Autodesk Fusion 360 part; units mm, degrees
sketch "M3 Standoff Profile" plane through (0, 0, 0) normal (0, 1, 0) x (1, 0, 0)
  arc A0 (-2.75, -1.3669) -> (-2.5588, -1.6981) centre (-2.3675, -1.3669) ccw
  arc A1 (0.1912, 3.065) -> (-0.1913, 3.065) centre (0, 2.7338) ccw
  arc A2 (-0.1912, -3.065) -> (0.1913, -3.065) centre (0, -2.7338) ccw
  arc A3 (2.5588, -1.6981) -> (2.75, -1.3669) centre (2.3675, -1.3669) ccw
  line L0 (2.75, -1.3669) -> (2.75, 1.3669)
  line L1 (-2.75, 1.3669) -> (-2.75, -1.3669)
  arc A4 (2.75, 1.3669) -> (2.5588, 1.6981) centre (2.3675, 1.3669) ccw
  line L2 (-0.1913, 3.065) -> (-2.5588, 1.6981)
  line L3 (2.5587, 1.6981) -> (0.1912, 3.065)
  line L4 (-2.5588, -1.6981) -> (-0.1912, -3.065)
  line L5 (0.1913, -3.065) -> (2.5588, -1.6981)
  arc A5 (-2.5588, 1.6981) -> (-2.75, 1.3669) centre (-2.3675, 1.3669) ccw
  line L6 (0, 2.7338) -> (0, -2.7338) construction
  dimension "d28" = 120
  dimension "d29" = 0.3825
  dimension "d30" = 2.75
  dimension "d31" = 5.5
  dimension "d32" = 120
extrude "Extrude1" add sketch "M3 Standoff Profile" along normal blind 20
hole "Hole1" at (0, 0, 0) direction (0, 1, 0) diameter 2.529 depth 8 tip angle 118
ref_plane "WorkPlane1" through (0, 10, 0) normal (0.5, 0, 0.866) x (0.866, 0, -0.5)
sketch "Sketch2" plane through (0, 0, 0) normal (0.5, 0, 0.866) x (0.866, 0, -0.5)
  line L0 (-3.065, 0) -> (-1.6981, 0)
  line L1 (-1.6981, 0) -> (-1.6981, 20)
  line L2 (-1.6981, 20) -> (-3.065, 20)
  line L3 (-3.065, 20) -> (-3.065, 0)
  line L4 (1.6981, 0) -> (3.065, 0)
  line L5 (3.065, 20) -> (1.6981, 20)
  line L6 (1.6981, 20) -> (1.6981, 0)
  line L7 (-3.065, 0) -> (-3.1163, 0)
  line L8 (-3.065, 0) -> (-3.065, 20)
  line L9 (-3.065, 20) -> (-3.1163, 20)
  line L10 (-3.065, 20) -> (-3.065, 0)
  line L11 (3.1163, 0) -> (3.065, 0)
  line L12 (3.1163, 20) -> (3.065, 20)
  line L13 (3.065, 20) -> (3.065, 0) construction
  line L14 (1.6981, 0) -> (1.3669, 0)
  line L15 (1.6981, 0) -> (1.6981, 20)
  line L16 (1.6981, 20) -> (1.3669, 20)
  line L17 (1.3669, 20) -> (1.3669, 0)
  line L18 (3.1163, 0) -> (3.1163, 0.25)
  line L19 (3.1163, 0) -> (2.8663, 0)
  line L20 (2.8663, 0) -> (3.1163, 0.25)
  line L21 (3.1163, 20) -> (2.8663, 20)
  line L22 (3.1163, 20) -> (3.1163, 19.75)
  line L23 (2.8663, 20) -> (3.1163, 19.75)
  dimension "d12" = 0.25
  dimension "d13" = 0.25
  dimension "d14" = 0.25
  dimension "d15" = 0.25
revolve "Revolve1" cut sketch "Sketch2" angle 360 about axis through (0, 1.75, 0) along (0, 1, 0) contours L4 L11 L18 L19 L20 | L5 L12 L21 L22 L23
sketch "Sketch3" plane through (0, 20, 0) normal (0, 1, 0) x (-1, 0, 0)
  arc A0 (-0.6752, -2.7856) -> (0.6752, -2.7856) centre (0, 0) ccw
  line L0 (0.6752, -2.7856) -> (2.0748, -1.9776)
  arc A1 (2.0748, -1.9776) -> (2.75, -0.808) centre (0, 0) ccw
  line L1 (2.75, -0.808) -> (2.75, 0.808)
  arc A2 (2.75, 0.808) -> (2.0748, 1.9776) centre (0, 0) ccw
  line L2 (2.0748, 1.9776) -> (0.6752, 2.7856)
  arc A3 (0.6752, 2.7856) -> (-0.6752, 2.7856) centre (0, 0) ccw
  line L3 (-0.6752, 2.7856) -> (-2.0748, 1.9776)
  arc A4 (-2.0748, 1.9776) -> (-2.75, 0.808) centre (0, 0) ccw
  line L4 (-2.75, 0.808) -> (-2.75, -0.808)
  arc A5 (-2.75, -0.808) -> (-2.0748, -1.9776) centre (0, 0) ccw
  line L5 (-2.0748, -1.9776) -> (-0.6752, -2.7856)
  circle A6 centre (0, 0) radius 1.5
  circle A7 centre (0, 0) radius 1.35
  dimension "d17" = 3
  dimension "d18" = 2.7
extrude "Extrude2" add sketch "Sketch3" along normal blind 0.75 contours A7
extrude "Extrude3" add sketch "Sketch3" along normal blind 4 from surface at 0.75 contours A6 | A7
fillet "Fillet1" radius 0.25 1 edges at (1.2586, 20, 0.4882)
chamfer "Chamfer3" distance 0.15 angle 45 2 edges at (1.3985, 20.75, -0.5424) (1.3985, 24.75, -0.5424)
chamfer "Chamfer3" distance 0.3 angle 45 1 edges at (0.4573, 0, 1.1789)
equation "Thread_Length = 4 mm"
equation "Spacing = 20 mm"
equation "d3 = Spacing"
equation "d22 = Thread_Length"
equation "d30 = Hex_Width / 2"
equation "d31 = d30 * 2"
equation "d32 = d28"
equation "Hex_Width = 5.5 mm"
properties part number "20-4 M-F Standoff"
Check sheet for the modelled part. Datum: model origin and axes. Units: mm. A direction names the side the tool comes from. Give positions to 0.01 mm unless a question says otherwise; leave off trailing zeros. Loops run counter-clockwise (first coordinate to the right, second up) from the corner with the lowest first, then second, coordinate; pieces in that order, holes last. Notation, with made-up numbers: M 56,-39.5 L 92,-39.5 A16 ccw 92,-12.5 Z; hole C 35,-33.75 d1. An arc over 180 degrees is marked long. Answer as a JSON object with one key per item and string values. Group by question number.
Q1. Cross-section at B-B on y = 17. Record the cut outline in (x, z) (3 decimals).
Q2. Material ranges on line 1 along X through (y, z) = (2, 0); line 2 along Z through (x, y) = (0, 3.5); line 3 along Y through (x, z) = (0.7, -2), recorded low to high. Write a range as [from, to].
Q3. Access from +Z, -Z, +X, -X, +Y, -Y to the whole of each face (thin tool, end or side, straight path). Record for faces 4 (the flat face through (-1.3, 0, 1.2)), 5 (the cylindrical face through (0.769, 4.204, 1.003)), 6 (the flat face through (-1.3, 20, 1.2)).
Q4. Release check for a two-part mould opening along Y. For faces 1 (the cylindrical face through (0.29, 20.5, 1.32)), 2 (the cylindrical face through (1.5, 22.72, -0.07)), 3 (the flat face through (0, 24.75, 0)) record: released by +Y, released by -Y, zero draft, split by the parting line, or undercut.
Q5. Go/stop test with a flat-tipped pin: P1, Ø1, axis at x = 0, z = -1, coming from the -Y side. Record where the tip stops, or that it passes through.
Evaluation:
{
 "1": {"outline": "M -2.75,-1.367 A0.382 ccw -2.559,-1.698 L -0.191,-3.065 A0.382 ccw 0.191,-3.065 L 2.559,-1.698 A0.382 ccw 2.75,-1.367 L 2.75,1.367 A0.382 ccw 2.559,1.698 L 0.191,3.065 A0.382 ccw -0.191,3.065 L -2.559,1.698 A0.382 ccw -2.75,1.367 Z"},
 "2": {"line 1": "x = [-2.75, -1.26], [1.26, 2.75]", "line 2": "z = [-3.12, -1.26], [1.26, 3.12]", "line 3": "y = [0, 20]"},
 "3": {"face 4": "+Z, -Z, +X, -X, -Y", "face 5": "-Y", "face 6": "+Y"},
 "4": {"face 1": "undercut", "face 2": "zero draft", "face 3": "released by +Y"},
 "5": {"P1": "stops at y = 0.06"}
}
